Here's how the part is built. I have some questions about the finished solid (model axes, mm). Coordinates: 2 decimals unless noted, no trailing zeros.
Item 1: Please list where these lines run through material, in increasing order: line 1 (Y direction, x = -94, z = 0.85); line 2 (X direction, y = -8, z = 0.15); line 3 (X direction, y = -13.5, z = 1.4).
Item 2: I want a section at A-A (z = 0.4). Count the separate pieces of the cut face and the enclosed holes in it, and give its area (3 significant figures).
Item 3: If we mould it in two halves opening along X, with no side actions, what happens to faces 1 (the face through (-2, 0, 0)), 2 (the face through (-123.16, -29.66, 0.91)), 3 (the face through (78.363, -2.928, 0.94))? For each: pulls with the +X half, pulls with the -X half, needs draft (parallel to the pull), parting line crosses it, or undercut.
Item 4: I'm going to push flat-ended pins straight in: P1, Ø4.5, axis at x = -119.89, y = 17.46, coming from the +Z side; P2, Ø0.6, axis at y = -7.5, z = 1, coming from the +X side; P3, Ø0.6, axis at y = 2.5, z = 1, coming from the -X side; P4, Ø0.9, axis at x = 124, z = 1.5, coming from the -Y side. Where does each tip first touch, or does it pass through?
from build123d import *

# Parameters (mm, degrees)
MAINBODY_DEPTH    = 1.8542
SKETCH3_R         = 1.9685
MOUNTHOLES_DEPTH  = 2.8542
PANELCUTOUT_REACH = 3.854
SKETCH4_R         = 2.667
SKETCH4_W         = 8.534035503
SKETCH4_H         = 3.447371256
SKETCH4_W_2       = 17.373674213
SKETCH4_H_2       = 9.779
SKETCH4_W_3       = 17.808
SKETCH4_H_3       = 7.758


with BuildPart() as part:
    # Sketch2 → MainBody (new body)
    with BuildSketch(Plane.XY):
        with BuildLine():
            Line((118.618, 31.5722), (-118.618, 31.5722))
            ThreePointArc((-118.618, 31.5722), (-123.108128061, 29.712328061), (-124.968, 25.2222))
            Line((-124.968, 25.2222), (-124.968, 9.9822))
            Line((-124.968, 9.9822), (-121.793, 9.9822))
            Line((-121.793, 9.9822), (-121.793, -9.9822))
            Line((-121.793, -9.9822), (-124.968, -9.9822))
            Line((-124.968, -9.9822), (-124.968, -25.2222))
            ThreePointArc((-124.968, -25.2222), (-123.108128061, -29.712328061), (-118.618, -31.5722))
            Line((-118.618, -31.5722), (118.618, -31.5722))
            ThreePointArc((118.618, -31.5722), (123.108128061, -29.712328061), (124.968, -25.2222))
            Line((124.968, -25.2222), (124.968, -9.9822))
            Line((124.968, -9.9822), (121.793, -9.9822))
            Line((121.793, -9.9822), (121.793, 9.9822))
            Line((121.793, 9.9822), (124.968, 9.9822))
            Line((124.968, 9.9822), (124.968, 25.2222))
            ThreePointArc((124.968, 25.2222), (123.108128061, 29.712328061), (118.618, 31.5722))
        make_face()
    extrude(amount=MAINBODY_DEPTH)

    # Sketch3 → MountHoles (cut, through all)
    with BuildSketch(Plane.XY.offset(1.8542)):
        with Locations((-119.888, 17.4625)):
            Circle(SKETCH3_R)
        with Locations((119.888, 17.4625)):
            Circle(SKETCH3_R)
        with Locations((119.888, -17.4625)):
            Circle(SKETCH3_R)
        with Locations((-119.888, -17.4625)):
            Circle(SKETCH3_R)
    extrude(amount=-MOUNTHOLES_DEPTH, mode=Mode.SUBTRACT)

    # Sketch4 → PanelCutout (cut, up to next)
    with BuildSketch(Plane.XY.offset(1.8542), mode=Mode.PRIVATE) as panelcutout_sk1:
        with Locations((90.297, -3.729450093)):
            Circle(SKETCH4_R)
    panelcutout_tool1 = extrude(panelcutout_sk1.sketch, amount=-PANELCUTOUT_REACH, mode=Mode.PRIVATE) & part.part
    add(panelcutout_tool1.solids().sort_by_distance((90.297, -3.72945, 1.8542))[0], mode=Mode.SUBTRACT)
    # Sketch4 → PanelCutout (cut, up to next)
    with BuildSketch(Plane.XY.offset(1.8542), mode=Mode.PRIVATE) as panelcutout_sk2:
        with Locations((75.819, -3.729450093)):
            Circle(SKETCH4_R)
    panelcutout_tool2 = extrude(panelcutout_sk2.sketch, amount=-PANELCUTOUT_REACH, mode=Mode.PRIVATE) & part.part
    add(panelcutout_tool2.solids().sort_by_distance((75.819, -3.72945, 1.8542))[0], mode=Mode.SUBTRACT)
    # Sketch4 → PanelCutout (cut, up to next)
    with BuildSketch(Plane.XY.offset(1.8542), mode=Mode.PRIVATE) as panelcutout_sk3:
        with Locations((102.1588002, 14.470550015)):
            Rectangle(SKETCH4_W, SKETCH4_H)
    panelcutout_tool3 = extrude(panelcutout_sk3.sketch, amount=-PANELCUTOUT_REACH, mode=Mode.PRIVATE) & part.part
    add(panelcutout_tool3.solids().sort_by_distance((102.1588, 14.47055, 1.8542))[0], mode=Mode.SUBTRACT)
    # Sketch4 → PanelCutout (cut, up to next)
    with BuildSketch(Plane.XY.offset(1.8542), mode=Mode.PRIVATE) as panelcutout_sk4:
        with Locations((-87.246762894, -6.11895)):
            Rectangle(SKETCH4_W_2, SKETCH4_H_2)
    panelcutout_tool4 = extrude(panelcutout_sk4.sketch, amount=-PANELCUTOUT_REACH, mode=Mode.PRIVATE) & part.part
    add(panelcutout_tool4.solids().sort_by_distance((-87.246763, -6.11895, 1.8542))[0], mode=Mode.SUBTRACT)
    # Sketch4 → PanelCutout (cut, up to next)
    with BuildSketch(Plane.XY.offset(1.8542), mode=Mode.PRIVATE) as panelcutout_sk5:
        with Locations((-62.3548, -7.00245)):
            Rectangle(SKETCH4_W_3, SKETCH4_H_3)
    panelcutout_tool5 = extrude(panelcutout_sk5.sketch, amount=-PANELCUTOUT_REACH, mode=Mode.PRIVATE) & part.part
    add(panelcutout_tool5.solids().sort_by_distance((-62.3548, -7.00245, 1.8542))[0], mode=Mode.SUBTRACT)
    # Sketch4 → PanelCutout (cut, up to next)
    with BuildSketch(Plane.XY.offset(1.8542), mode=Mode.PRIVATE) as panelcutout_sk6:
        Polygon((-36.424791576, -11.38945), (-36.424791576, 1.12655), (-48.968754151, 1.12655), (-48.968754151, -11.38945), (-51.1788, -11.38945), (-51.1788, -17.73945), (-34.1608, -17.73945), (-34.1608, -11.38945), align=None)
    panelcutout_tool6 = extrude(panelcutout_sk6.sketch, amount=-PANELCUTOUT_REACH, mode=Mode.PRIVATE) & part.part
    add(panelcutout_tool6.solids().sort_by_distance((-42.685776, -8.977195, 1.8542))[0], mode=Mode.SUBTRACT)
    # Sketch4 → PanelCutout (cut, up to next)
    with BuildSketch(Plane.XY.offset(1.8542), mode=Mode.PRIVATE) as panelcutout_sk7:
        Polygon((60.2488, 6.547255322), (60.2488, 1.946245078), (60.577194878, 1.6178502), (66.168805122, 1.6178502), (66.4972, 1.946245078), (66.4972, 6.547255322), (66.168805122, 6.8756502), (60.577194878, 6.8756502), align=None)
    panelcutout_tool7 = extrude(panelcutout_sk7.sketch, amount=-PANELCUTOUT_REACH, mode=Mode.PRIVATE) & part.part
    add(panelcutout_tool7.solids().sort_by_distance((63.373, 4.24675, 1.8542))[0], mode=Mode.SUBTRACT)
    # Sketch4 → PanelCutout (cut, up to next)
    with BuildSketch(Plane.XY.offset(1.8542), mode=Mode.PRIVATE) as panelcutout_sk8:
        Polygon((99.3648, 6.547255322), (99.3648, 1.946245078), (99.693194878, 1.6178502), (105.284805122, 1.6178502), (105.6132, 1.946245078), (105.6132, 6.547255322), (105.284805122, 6.8756502), (99.693194878, 6.8756502), align=None)
    panelcutout_tool8 = extrude(panelcutout_sk8.sketch, amount=-PANELCUTOUT_REACH, mode=Mode.PRIVATE) & part.part
    add(panelcutout_tool8.solids().sort_by_distance((102.489, 4.24675, 1.8542))[0], mode=Mode.SUBTRACT)


solid = part.part
Answer:
1. line 1: y = -31.57 to -11.01, -1.23 to 31.57
1. line 2: x = -121.79 to -95.93, -78.56 to -71.26, -53.45 to -48.97, -36.42 to 121.79
1. line 3: x = -124.97 to -51.18, -34.16 to 124.97
2. separate pieces: 1
2. enclosed holes: 12
2. area: 14,900 mm2
3. face 1: needs draft
3. face 2: pulls with the -X half
3. face 3: undercut
4. P1: stops at z = 1.85
4. P2: stops at x = 121.79
4. P3: stops at x = -121.79
4. P4: stops at y = -29.22
